```python
from build123d import *

# Parameters (mm, degrees)
EXTRUDE_1_DEPTH     = 17.5
SKETCH_3_W          = 24
SKETCH_3_H          = 9
SKETCH_3_R          = 3.5
CUT_EXTRUDE_1_DEPTH = 4
SKETCH_6_R          = 4
CUT_EXTRUDE_2_DEPTH = 8.85
SKETCH_7_R          = 4
CUT_EXTRUDE_3_DEPTH = 4.75
SKETCH_9_W          = 7.2
SKETCH_9_H          = 1.5
CUT_EXTRUDE_5_DEPTH = 1
FILLET_1_R          = 0.5
SKETCH_8_R          = 0.75
CUT_EXTRUDE_4_DEPTH = 38.428601697


with BuildPart() as part:
    # Эскиз1 → Бобышка-Вытянуть1 (new, symmetric)
    with BuildSketch(Plane(origin=(0, 0, 0), x_dir=(0, 0, -1), z_dir=(1, 0, 0))):
        with BuildLine():
            Line((-7.765, 7), (7.765, 7))
            ThreePointArc((7.765, 7), (11.265, 3.5), (7.765, 0))
            Line((7.765, 0), (-7.765, 0))
            ThreePointArc((-7.765, 0), (-11.265, 3.5), (-7.765, 7))
        make_face()
    extrude(amount=EXTRUDE_1_DEPTH, both=True)

    # Эскиз3 → Вырез-Вытянуть1 (cut)
    with BuildSketch(Plane(origin=(17.5, 0, 0), x_dir=(0, 0, -1), z_dir=(1, 0, 0))):
        with Locations((0, 3.5)):
            Rectangle(SKETCH_3_W, SKETCH_3_H)
        with Locations(Location((-7.765, 3.5, 0), (0, 0, 90))):
            Circle(SKETCH_3_R, mode=Mode.SUBTRACT)
    cut_extrude_1 = extrude(amount=-CUT_EXTRUDE_1_DEPTH, mode=Mode.SUBTRACT)

    # Зеркальное отражение1: Вырез-Вытянуть1 across plane
    add(cut_extrude_1.mirror(Plane(origin=(0, 0, 0), x_dir=(0, 0, 1), z_dir=(1, 0, 0))), mode=Mode.SUBTRACT)

    # Эскиз6 → Вырез-Вытянуть2 (cut, symmetric)
    with BuildSketch(Plane(origin=(0, 0, 0), x_dir=(0, 0, -1), z_dir=(1, 0, 0))):
        with Locations((-7.765, 3.5)):
            Circle(SKETCH_6_R)
    extrude(amount=CUT_EXTRUDE_2_DEPTH, both=True, mode=Mode.SUBTRACT)

    # Эскиз7 → Вырез-Вытянуть3 (cut)
    with BuildSketch(Plane(origin=(13.5, 0, 0), x_dir=(0, 0, -1), z_dir=(1, 0, 0))):
        with Locations((7.765, 3.5)):
            Circle(SKETCH_7_R)
    cut_extrude_3 = extrude(amount=-CUT_EXTRUDE_3_DEPTH, mode=Mode.SUBTRACT)

    # Эскиз9 → Вырез-Вытянуть5 (cut)
    with BuildSketch(Plane(origin=(17.5, 0, 0), x_dir=(0, 0, -1), z_dir=(1, 0, 0))):
        with Locations((-7.765, 3.5)):
            Rectangle(SKETCH_9_W, SKETCH_9_H)
    cut_extrude_5 = extrude(amount=-CUT_EXTRUDE_5_DEPTH, mode=Mode.SUBTRACT)

    # Зеркальное отражение2: Вырез-Вытянуть3, Вырез-Вытянуть5 across plane
    add(cut_extrude_3.mirror(Plane(origin=(0, 0, 0), x_dir=(0, 0, 1), z_dir=(1, 0, 0))), mode=Mode.SUBTRACT)
    add(cut_extrude_5.mirror(Plane(origin=(0, 0, 0), x_dir=(0, 0, 1), z_dir=(1, 0, 0))), mode=Mode.SUBTRACT)

    # Скругление1
    fillet_1_edges = [part.edges().sort_by_distance(p)[0] for p in [
        (-11.125, 0, -5.828508327),
        (-11.125, 7, -5.828508327),
        (0, 7, 5.828508327),
        (0, 0, 5.828508327),
        (11.125, 0, -5.828508327),
        (11.125, 7, -5.828508327),
    ]]
    fillet(fillet_1_edges, radius=FILLET_1_R)

    # Эскиз8 → Вырез-Вытянуть4 (cut, through all)
    with BuildSketch(Plane(origin=(17.5, 0, 0), x_dir=(0, 0, -1), z_dir=(1, 0, 0))):
        with Locations((-7.765, 3.5)):
            Circle(SKETCH_8_R)
        with Locations((7.765, 3.5)):
            Circle(SKETCH_8_R)
    extrude(amount=-CUT_EXTRUDE_4_DEPTH, mode=Mode.SUBTRACT)


solid = part.part
```
Check sheet for the modelled part. Datum: model origin and axes. Units: mm. A direction names the side the tool comes from. Round coordinates to 2 decimals unless told otherwise and drop trailing zeros. Loops run counter-clockwise (first coordinate to the right, second up) from the corner with the lowest first, then second, coordinate; pieces in that order, holes last. Notation, with made-up numbers: (2, 57.25) -> (17, 57.25) arc R13 ccw to (17, 74.25) -> close; hole circle Ø2 at (80.5, 51.25). An arc over 180 degrees is marked (long way). Answer in a Markdown table with one row per item.
Q1. Set-up check for faces 5 (the face through (0.124, 0.289, 4.864)), 6 (the face through (11.158, 0.289, -4.864)), 7 (the face through (-11.158, 0.289, -4.864)): record each of +Z, -Z, +X, -X, +Y, -Y from which the full face is reachable in a straight line by a thin tool's end or side.
Data:
| item | result |
|---|---|
| face 5 | +Z |
| face 6 | -Z, +X |
| face 7 | -Z, -X |
Q2. Thickness scan on L1, parallel to X at y = 3.25, z = 6.5; L2, parallel to X at y = 5, z = 9.25; L3, parallel to Z at x = -12.5, y = 3.5 (3 decimals). Record the ranges inside material, lowest first.
Data:
| item | result |
|---|---|
| L1 | x = -16.5 to -8.85, 8.85 to 16.5 |
| L2 | x = -17.5 to -8.85, 8.85 to 17.5 |
| L3 | z = -3.765 to 7.015, 8.515 to 11.265 |
Q3. Sectioned sample at B-B on z = 9. Enter the section's corners in (x, y).
Data:
| item | result |
|---|---|
| outline | (-17.5, 0.23) -> (-8.85, 0.23) -> (-8.85, 6.77) -> (-17.5, 6.77) -> (-17.5, 4.25) -> (-16.5, 4.25) -> (-16.5, 2.75) -> (-17.5, 2.75) -> close; (8.85, 0.23) -> (17.5, 0.23) -> (17.5, 2.75) -> (16.5, 2.75) -> (16.5, 4.25) -> (17.5, 4.25) -> (17.5, 6.77) -> (8.85, 6.77) -> close |
Q4. Sectioned sample at A-A on x = -13. Enter the section's corners in (y, z) (3 decimals), then the cut area to 3 significant figures.
Data:
| item | result |
|---|---|
| outline | (0, -4.411) arc R0.5 ccw to (0.833, -4.784) arc R4 cw to (6.167, -4.784) arc R0.5 ccw to (7, -4.411) -> (7, 7.765) arc R3.5 ccw to (0, 7.765) -> close; hole circle Ø1.5 at (3.5, 7.765) |
| area | 102 mm^2 |
Q5. Release check for a two-part mould opening along X. For faces 1 (the face through (-16.5, 4, 6)), 2 (the face through (12.729, 3.044, 8.36)), 3 (the face through (-8.85, 4, 7)), 4 (the face through (16.5, 4, 6)) record: released by +X, released by -X, zero draft, split by the parting line, or undercut.
Data:
| item | result |
|---|---|
| face 1 | released by -X |
| face 2 | zero draft |
| face 3 | undercut |
| face 4 | released by +X |
Q6. Go/stop test with flat-tipped pins: P1, Ø0.8, axis at x = 17, z = 9, coming from the +Y side; P2, Ø4, axis at x = 6.5, z = 9, coming from the +Y side; P3, Ø0.8, axis at y = 3.5, z = 9, coming from the -X side; P4, Ø1.2, axis at y = 3.5, z = 6, coming from the +X side. Record where each tip stops, or that it passes through.
Data:
| item | result |
|---|---|
| P1 | stops at y = 6.9 |
| P2 | passes through |
| P3 | stops at x = -16.5 |
| P4 | stops at x = 16.5 |
Q7. Sectioned sample at D-D on y = 1.75. Enter the section's corners in (x, z), then the cut area to 3 significant figures.
Data:
| item | result |
|---|---|
| outline | (-17.5, 4.73) -> (-13.5, 4.73) -> (-13.5, -4.17) -> (-8.75, -4.17) -> (-8.75, -10.8) -> (8.75, -10.8) -> (8.75, -4.17) -> (13.5, -4.17) -> (13.5, 4.73) -> (17.5, 4.73) -> (17.5, 10.8) -> (8.85, 10.8) -> (8.85, 4.17) -> (-8.85, 4.17) -> (-8.85, 10.8) -> (-17.5, 10.8) -> close |
| area | 451 mm^2 |
Q8. Sectioned sample at C-C on y = 3.5. Enter the section's corners in (x, z) (3 decimals).
Data:
| item | result |
|---|---|
| outline | (-16.5, 4.265) -> (-13.5, 4.265) -> (-13.5, -3.765) -> (-8.75, -3.765) -> (-8.75, -7.015) -> (8.75, -7.015) -> (8.75, -3.765) -> (13.5, -3.765) -> (13.5, 4.265) -> (16.5, 4.265) -> (16.5, 7.015) -> (8.85, 7.015) -> (8.85, 3.765) -> (-8.85, 3.765) -> (-8.85, 7.015) -> (-16.5, 7.015) -> close; (-16.5, 8.515) -> (-8.85, 8.515) -> (-8.85, 11.265) -> (-16.5, 11.265) -> close; (-8.75, -11.265) -> (8.75, -11.265) -> (8.75, -8.515) -> (-8.75, -8.515) -> close; (8.85, 8.515) -> (16.5, 8.515) -> (16.5, 11.265) -> (8.85, 11.265) -> close |
